from build123d import *

# Parameters (mm, degrees)
BOSS_EXTRUDE1_DEPTH            = 2
BOSS_EXTRUDE2_DEPTH            = 10
CUT_EXTRUDE1_START             = 10
CUT_EXTRUDE1_DEPTH             = 4
CUT_EXTRUDE2_START             = 10
SKETCH1_5_R                    = 11
CUT_EXTRUDE2_DEPTH             = 4
F_14_25_14_25_DIAMETER_HOLE1_D = 14.25
F_5_0_5_DIAMETER_HOLE1_D       = 5
F_5_0_5_DIAMETER_HOLE1_DEPTH   = 10
F_10_2_10_2_DIAMETER_HOLE1_D   = 10.2
EXTRUDE_THIN1_START            = 12
SKETCH1_6_R                    = 14
SKETCH1_6_R_2                  = 11
EXTRUDE_THIN1_DEPTH            = 2
SKETCH8_W                      = 1.15
SKETCH8_H                      = 11.65
SKETCH8_W_2                    = 4
SKETCH8_H_2                    = 12
FILLET1_R                      = 0.5
FILLET2_R                      = 5
FILLET3_R                      = 0.25
CUT_EXTRUDE_THIN1_START        = -2
CUT_EXTRUDE_THIN1_DEPTH        = 1
F_3_0_3_DIAMETER_HOLE1_D       = 3
F_3_0_3_DIAMETER_HOLE1_DEPTH   = 2
F_3_0_3_DIAMETER_HOLE1_TIP     = 0.901290929


with BuildPart() as part:
    # Sketch1 → Boss-Extrude1 (new body)
    with BuildSketch(Plane.XY):
        Polygon((15, 45), (-15, 45), (-35, 40), (-35, 25), (-37, 25), (-37, -25), (-35, -25), (-35, -40), (-15, -45), (15, -45), (35, -40), (35, -25), (37, -25), (37, 25), (35, 25), (35, 40), align=None)
    extrude(amount=-BOSS_EXTRUDE1_DEPTH)

    # Sketch1<3> → Boss-Extrude2 (add)
    with BuildSketch(Plane.XY):
        with BuildLine():
            Line((32, 50), (-32, 50))
            ThreePointArc((-32, 50), (-37.656854249, 47.656854249), (-40, 42))
            Line((-40, 42), (-40, -42))
            ThreePointArc((-40, -42), (-37.656854249, -47.656854249), (-32, -50))
            Line((-32, -50), (32, -50))
            ThreePointArc((32, -50), (37.656854249, -47.656854249), (40, -42))
            Line((40, -42), (40, 42))
            ThreePointArc((40, 42), (37.656854249, 47.656854249), (32, 50))
        make_face()
    extrude(amount=BOSS_EXTRUDE2_DEPTH)

    # Sketch1<4> → Cut-Extrude1 (cut)
    with BuildSketch(Plane.XY.offset(CUT_EXTRUDE1_START)):
        with BuildLine():
            Line((33, -7), (41, -7))
            ThreePointArc((41, -7), (49, -15), (41, -23))
            Line((41, -23), (33, -23))
            ThreePointArc((33, -23), (25, -15), (33, -7))
        make_face()
        with BuildLine():
            Line((-33, -7), (-41, -7))
            ThreePointArc((-41, -7), (-49, -15), (-41, -23))
            Line((-41, -23), (-33, -23))
            ThreePointArc((-33, -23), (-25, -15), (-33, -7))
        make_face()
    extrude(amount=-CUT_EXTRUDE1_DEPTH, mode=Mode.SUBTRACT)

    # Sketch1<5> → Cut-Extrude2 (cut)
    with BuildSketch(Plane.XY.offset(CUT_EXTRUDE2_START)):
        with Locations(Location((0, -15, 0), (0, 0, 180))):
            Circle(SKETCH1_5_R)
    extrude(amount=-CUT_EXTRUDE2_DEPTH, mode=Mode.SUBTRACT)

    # Ø14.25 (14.25) Diameter Hole1 (through all)
    with Locations(Plane.XY.offset(10)):
        with Locations((0, -15)):
            Hole(F_14_25_14_25_DIAMETER_HOLE1_D / 2)

    # Ø5.0 (5) Diameter Hole1
    with Locations(Plane.XY.offset(10)):
        with Locations((-33.753049524, 42.191311906), (33.753049524, 42.191311906), (33.753049524, -42.191311906), (-33.753049524, -42.191311906)):
            Hole(F_5_0_5_DIAMETER_HOLE1_D / 2, depth=F_5_0_5_DIAMETER_HOLE1_DEPTH)

    # Ø10.2 (10.2) Diameter Hole1 (through all)
    with Locations(Plane.XY.offset(10)):
        with Locations((-25, 29), (25, 29), (25, -29), (-25, -29)):
            Hole(F_10_2_10_2_DIAMETER_HOLE1_D / 2)

    # Sketch1<6> → Extrude-Thin1 (add)
    with BuildSketch(Plane.XY.offset(EXTRUDE_THIN1_START)):
        with Locations((0, -15)):
            Circle(SKETCH1_6_R)
        with Locations((0, -15)):
            Circle(SKETCH1_6_R_2, mode=Mode.SUBTRACT)
    extrude(amount=-EXTRUDE_THIN1_DEPTH)

    # Sketch8 → Cut-Revolve1 (revolve, cut)
    with BuildSketch(Plane(origin=(0, 0, 0), x_dir=(0, 0, -1), z_dir=(1, 0, 0)), mode=Mode.PRIVATE) as cut_revolve1_sk:
        with Locations((-10.425, -9.175)):
            Rectangle(SKETCH8_W, SKETCH8_H)
        with Locations((-6.35, -9)):
            Rectangle(SKETCH8_W_2, SKETCH8_H_2)
    revolve(cut_revolve1_sk.sketch.rotate(Axis((0, -15, 0), (0, 0, 1)), 270), axis=Axis((0, -15, 0), (0, 0, 1)), mode=Mode.SUBTRACT)

    # Fillet1
    fillet1_edges = [part.edges().sort_by_distance(p)[0] for p in [
        (-35, 25, -1),
        (35, 25, -1),
        (37, 25, -1),
        (37, -25, -1),
        (35, -25, -1),
        (-35, -25, -1),
        (-37, -25, -1),
        (-37, 25, -1),
    ]]
    fillet(fillet1_edges, radius=FILLET1_R)

    # Fillet2
    # the kernel refuses this fillet: 5 mm, written as the material it takes off along each edge
    with BuildSketch(Plane(origin=(-35, 40, 0), x_dir=(0.970142500145332, 0.24253562503633277, 0), z_dir=(0, 0, -1)), Plane(origin=(35, 40, 0), x_dir=(0, -1, 0), z_dir=(0, 0, -1))) as fillet2_piece_1:
        with BuildLine():
            CenterArc((FILLET2_R * 0.780776406404, FILLET2_R), FILLET2_R, 194.036243468, 75.963756532)
            Line((-FILLET2_R * 0.189366093741, FILLET2_R * 0.757464374964), (0, 0))
            Line((0, 0), (FILLET2_R * 0.780776406404, 0))
        make_face()
    extrude(amount=11.75970508, mode=Mode.SUBTRACT)
    with BuildSketch(Plane(origin=(-15, 45, 0), x_dir=(1, 0, 0), z_dir=(0, 0, -1)), Plane(origin=(15, 45, 0), x_dir=(0.9701425001453312, -0.2425356250363357, 0), z_dir=(0, 0, -1))) as fillet2_piece_2:
        with BuildLine():
            CenterArc((FILLET2_R * 0.123105625618, FILLET2_R), FILLET2_R, 255.963756532, 14.036243468)
            Line((-FILLET2_R * 0.119429999419, FILLET2_R * 0.0298574998547), (0, 0))
            Line((0, 0), (FILLET2_R * 0.123105625618, 0))
        make_face()
    extrude(amount=3.53882032, mode=Mode.SUBTRACT)
    with BuildSketch(Plane(origin=(35, -40, 0), x_dir=(0, 1, 0), z_dir=(0, 0, -1)), Plane(origin=(-35, -40, 0), x_dir=(0.9701425001453319, -0.24253562503633297, 0), z_dir=(0, 0, -1))) as fillet2_piece_3:
        with BuildLine():
            CenterArc((FILLET2_R * 0.780776406404, -FILLET2_R), FILLET2_R, 90, 75.963756532)
            Line((-FILLET2_R * 0.189366093741, -FILLET2_R * 0.757464374964), (0, 0))
            Line((0, 0), (FILLET2_R * 0.780776406404, 0))
        make_face()
    extrude(amount=11.75970508, mode=Mode.SUBTRACT)
    with BuildSketch(Plane(origin=(15, -45, 0), x_dir=(0.9701425001453312, 0.2425356250363357, 0), z_dir=(0, 0, -1)), Plane(origin=(-15, -45, 0), x_dir=(1, 0, 0), z_dir=(0, 0, -1))) as fillet2_piece_4:
        with BuildLine():
            CenterArc((FILLET2_R * 0.123105625618, -FILLET2_R), FILLET2_R, 90, 14.036243468)
            Line((-FILLET2_R * 0.119429999419, -FILLET2_R * 0.0298574998547), (0, 0))
            Line((0, 0), (FILLET2_R * 0.123105625618, 0))
        make_face()
    extrude(amount=3.53882032, mode=Mode.SUBTRACT)

    # Fillet3
    fillet3_edges = [part.edges().sort_by_distance(p)[0] for p in [
        (23.404914061, 42.898771485, 0),
        (0, 45, 0),
        (-23.404914061, 42.898771485, 0),
        (31.442974512, 40.883374443, 0),
        (14.99538819, 44.962537783, 0),
        (-14.99538819, 44.962537783, 0),
        (-31.442974512, 40.883374443, 0),
        (37.656854249, 47.656854249, 10),
        (0, 50, 0),
        (-37.656854249, 47.656854249, 0),
        (-40, 0, 0),
        (-37.656854249, -47.656854249, 10),
        (0, -50, 10),
        (37.656854249, -47.656854249, 10),
        (40, 17.5, 10),
        (0, 50, 10),
        (-37.656854249, 47.656854249, 10),
        (-40, 17.5, 10),
        (37.656854249, 47.656854249, 0),
        (40, 0, 0),
        (37.656854249, -47.656854249, 0),
        (0, -50, 0),
        (-37.656854249, -47.656854249, 0),
        (-40, -32.5, 10),
        (40, -32.5, 10),
    ]]
    fillet(fillet3_edges, radius=FILLET3_R)

    # Sketch1<8> → Cut-Extrude-Thin1 (cut)
    with BuildSketch(Plane.XY.offset(CUT_EXTRUDE_THIN1_START)):
        with BuildLine():
            Line((22, 15), (22, -15))
            ThreePointArc((22, -15), (0, -37), (-22, -15))
            Line((-22, -15), (-22, 15))
            ThreePointArc((-22, 15), (0, 37), (22, 15))
        make_face()
        with BuildLine():
            Line((20, 15), (20, -15))
            ThreePointArc((20, -15), (0, -35), (-20, -15))
            Line((-20, -15), (-20, 15))
            ThreePointArc((-20, 15), (0, 35), (20, 15))
        make_face(mode=Mode.SUBTRACT)
    extrude(amount=CUT_EXTRUDE_THIN1_DEPTH, mode=Mode.SUBTRACT)

    # Ø3.0 (3) Diameter Hole1
    with Locations(Plane(origin=(0, 0, -2), x_dir=(-1, 0, 0), z_dir=(0, 0, -1))):
        with Locations((0, 40), (0, -40)):
            Hole(F_3_0_3_DIAMETER_HOLE1_D / 2, depth=F_3_0_3_DIAMETER_HOLE1_DEPTH)
            with Locations((0, 0, -(F_3_0_3_DIAMETER_HOLE1_DEPTH + F_3_0_3_DIAMETER_HOLE1_TIP / 2))):  # 118° drill point
                Cone(0, F_3_0_3_DIAMETER_HOLE1_D / 2, F_3_0_3_DIAMETER_HOLE1_TIP, mode=Mode.SUBTRACT)


solid = part.part
Geometry: final body of the model. Coordinates: model frame, mm. A direction names the side the tool comes from. Give positions to 0.01 mm unless a question says otherwise; leave off trailing zeros. Order: outer loops, then holes, each group sorted by start corner. A loop starts at its lowest first (then second) coordinate and runs counter-clockwise, first axis right, second up. Notation, with made-up numbers: (3.25, -2) - (17.25, -2) arc R30 ccw to (17.25, 33) - close; hole circle Ø8 at (68.25, 14). An arc over 180 degrees is marked (long way). Use CSV: the item, a comma, the result in double quotes.
1. Section query B-B (z = 2.5). Give the number of separate pieces and of enclosed holes in the cut face, plus the area to 3 significant figures.
Answers below:
separate pieces,"1"
enclosed holes,"9"
area,"7,380 mm2"
2. Contact query for flat-ended pins moving along their axis: pin 1 (4 mm diameter, centred on y = -18.5, z = 0, fed in from +X); pin 2 (3 mm diameter, centred on x = 14, y = -5.5, fed in from +Z); pin 3 (4.5 mm diameter, centred on x = -33.75, y = -42.19, fed in from +Z); pin 4 (0.5 mm diameter, centred on x = 36, z = -0.5, fed in from -Y). Output: stop coordinate, or through.
Answers below:
pin 1,"x = 40"
pin 2,"z = 10"
pin 3,"z = 0"
pin 4,"y = -25"
3. Access query for faces 4 (the face through (37, 0, -1)), 5 (the face through (-37, -23, 8)), 6 (the face through (33, -15, 6)). Directions: +Z, -Z, +X, -X, +Y, -Y. A direction counts if a zero-diameter tool reaches every point of the face in a straight line with its end or side. Return the directions, or none.
Answers below:
face 4,"-Z, +X, +Y, -Y"
face 5,"+Z, -X"
face 6,"+Z, +X"
4. Mould query, pull axis Z, two halves, no side actions, for faces 1 (the face through (-20.95, -32.1, 3.92)), 2 (the face through (-1.56, -3.1, 6.32)), 3 (the face through (-33, -15, 6)). Classes: +Z half, -Z half, draft (parallel to the pull), parting line (faces both ways), or undercut.
Answers below:
face 1,"draft"
face 2,"undercut"
face 3,"+Z half"
5. Section query A-A (y = 29). Output: boundary loops of the cut face in (x, z), plus the area to 3 significant figures.
Answers below:
outline,"(-40, 0.25) arc R0.25 ccw to (-39.75, 0) - (-35, 0) - (-35, -2) - (-30.1, -2) - (-30.1, 10) - (-39.75, 10) arc R0.25 ccw to (-40, 9.75) - close; (-19.9, -2) - (-16.97, -2) - (-16.97, -1) - (-14.28, -1) - (-14.28, -2) - (14.28, -2) - (14.28, -1) - (16.97, -1) - (16.97, -2) - (19.9, -2) - (19.9, 10) - (-19.9, 10) - close; (30.1, -2) - (35, -2) - (35, 0) - (39.75, 0) arc R0.25 ccw to (40, 0.25) - (40, 9.75) arc R0.25 ccw to (39.75, 10) - (30.1, 10) - close"
area,"690 mm2"
6. Material intervals for line 1 along Y through (x, z) = (0, -0.75) (3 decimals); line 2 along Y through (x, z) = (-26, -1.5); line 3 along Y through (x, z) = (21, 6.25), sorted ascending. Write a range as from..to.
Answers below:
line 1,"-45..-41.5, -38.5..-22.125, -7.875..38.5, 41.5..45"
line 2,"-42.25..-34, -24..24, 34..42.25"
line 3,"-50..-32.16, -25.84..25.84, 32.16..50"
